Autodesk Inventor part; units mm, degrees
ref_plane "YZ Plane" through (0, 0, 0) normal (1, 0, 0) x (0, 1, 0)
ref_plane "XZ Plane" through (0, 0, 0) normal (0, 1, 0) x (-1, 0, 0)
ref_plane "XY Plane" through (0, 0, 0) normal (0, 0, 1) x (1, 0, 0)
sketch "Sketch_1" plane through (0, 0, 0) normal (0, 0, 1) x (1, 0, 0)
  line L0 (22.5, 0) -> (0, 0)
  line L1 (-22.5, 7.1) -> (-22.5, 6.15)
  line L2 (-22.5, 6.15) -> (-22.45, 6.15)
  line L3 (-22.45, 6.15) -> (-22.45, 6.1)
  line L4 (-22.45, 6.1) -> (22.45, 6.1)
  line L5 (22.45, 6.1) -> (22.45, 6.15)
  line L6 (22.45, 6.15) -> (22.5, 6.15)
  line L7 (22.5, 6.15) -> (22.5, 7.1)
  arc A0 (22.5, 7.1) -> (22.1, 7.5) centre (22.1, 7.1) ccw
  line L8 (22.1, 7.5) -> (17.5, 7.5)
  line L9 (17.5, 7.5) -> (17.5, 7.15)
  line L10 (17.5, 7.15) -> (16.4, 7.15)
  line L11 (16.4, 7.15) -> (16.4, 7.5)
  line L12 (16.4, 7.5) -> (-16.4, 7.5)
  line L13 (-16.4, 7.5) -> (-16.4, 7.15)
  line L14 (-16.4, 7.15) -> (-17.5, 7.15)
  line L15 (-17.5, 7.15) -> (-17.5, 7.5)
  line L16 (-17.5, 7.5) -> (-22.1, 7.5)
  arc A1 (-22.1, 7.5) -> (-22.5, 7.1) centre (-22.1, 7.1) ccw
revolve "Revolution1" add sketch "Sketch_1" angle 360 about axis through (22.5, 0, 0) along (1, 0, 0)
sketch "Sketch_3" plane through (0, 0, 0) normal (0, 0, 1) x (1, 0, 0)
  line L0 (22.5, 0) -> (0, 0)
  line L1 (-22.5, 6.1) -> (-22.5, 4)
  line L2 (-22.5, 4) -> (22.5, 4)
  line L3 (22.5, 4) -> (22.5, 6.1)
  line L4 (22.5, 6.1) -> (-22.5, 6.1)
revolve "Revolution2" add sketch "Sketch_3" angle 360 about axis through (22.5, 0, 0) along (1, 0, 0)
properties part number "C-LMUW8"
The listing builds one solid part. Answer for the finished solid, in the listing's coordinates (mm). A direction names the side the tool comes from. Coordinates: 2 decimals unless noted, no trailing zeros. Write each loop counter-clockwise with the first axis right and the second up, starting at its lowest first coordinate (ties: lowest second). Pieces come first, ordered by that corner, then holes.
Q1. Which of the six approach directions +Z, -Z, +X, -X, +Y, -Y give full straight-line access (tool end or side, diameter ignored) to faces 4 (the cylindrical face through (-0.23, -7.493, -0.33)), 5 (the cylindrical face through (-16.96, -0.93, -7.09))?
Returned:
face 4: +X, -X
face 5: none
Q2. Section A-A, the plane x = -0.5 is taken. Write down the section's boundary in (y, z), then the cut area to 3 significant figures.
Returned:
outline: circle Ø15 at (0, 0); hole circle Ø8 at (0, 0)
area: 126 mm2
Q3. Find the intervals of material crossed by line 1 along Z through (x, y) = (-6.5, 0); line 2 along Y through (x, z) = (13.5, 0.25); line 3 along X through (y, z) = (-5, -5.5), in increasing order.
Returned:
line 1: z = -7.5 to -4, 4 to 7.5
line 2: y = -7.5 to -3.99, 3.99 to 7.5
line 3: x = -22.32 to -17.5, -16.4 to 16.4, 17.5 to 22.32
Q4. The mould has two halves that part along X. Classify faces 1 (the flat face through (-22.5, 4, -1.3)), 2 (the flat face through (22.5, -2, 6)), 3 (the cylindrical face through (16.94, -0.93, -7.09)): released by +X, released by -X, zero draft, split by the parting line, or undercut.
Returned:
face 1: released by -X
face 2: released by +X
face 3: undercut
Q5. Given P1, Ø1, axis at x = 5, z = 2.5, coming from the -Y side; P2, Ø4, axis at x = -1.5, z = -5.5, coming from the -Y side; P3, Ø1, axis at x = 14.5, y = 5.5, coming from the -Z side, each flat-ended and moving along its own axis, determine where each tip first touches the part or whether it passes through.
Returned:
P1: stops at y = -7.23
P2: stops at y = -6.63
P3: stops at z = -5.59
